The listing builds one solid part. Answer for the finished solid, in the listing's coordinates (mm). A direction names the side the tool comes from. Round coordinates to 2 decimals unless told otherwise and drop trailing zeros. Write each loop counter-clockwise with the first axis right and the second up, starting at its lowest first coordinate (ties: lowest second). Pieces come first, ordered by that corner, then holes.
Autodesk Inventor part; units mm, degrees
ref_plane "YZ Plane" through (0, 0, 0) normal (1, 0, 0) x (0, 1, 0)
ref_plane "XZ Plane" through (0, 0, 0) normal (0, 1, 0) x (-1, 0, 0)
ref_plane "XY Plane" through (0, 0, 0) normal (0, 0, 1) x (1, 0, 0)
sketch "Sketch4" plane through (0, 0, 0) normal (0, 0, 1) x (1, 0, 0)
  line L0 (0, 0) -> (0, 60.2234)
  line L1 (0, 60.2234) -> (25.4, 60.2234)
  line L2 (25.4, 60.2234) -> (25.4, 53.8734)
  line L3 (25.4, 53.8734) -> (0, 53.8734)
  line L4 (0, 60.2234) -> (-12.7, 60.2234)
  line L5 (-12.7, 60.2234) -> (-12.7, 0)
  line L6 (-12.7, 0) -> (0, 0)
  dimension "d25" = 60.2234
  dimension "d26" = 6.35
  dimension "d27" = 25.4
  dimension "d28" = 12.7
extrude "Extrusion3" add sketch "Sketch4" along normal blind 25.4
sketch "Sketch5" plane through (-12.7, 60.2234, 0) normal (0, 1, 0) x (1, 0, 0)
  line L0 (38.1, 0) -> (38.1, -25.4)
  line L1 (38.1, -25.4) -> (0, -25.4)
  point P0 (25.4, -12.7)
  point P1 (15.621, -11.3751)
  point P2 (17.5484, -18.678)
  point P3 (24.0751, -22.479)
  point P4 (31.378, -20.5516)
  point P5 (35.179, -14.0249)
  point P6 (33.2516, -6.722)
  point P7 (26.7249, -2.921)
  point P8 (19.422, -4.8484)
  dimension "d36" = 360
  dimension "d45" = 9.779
  dimension "d46" = 12.7
  dimension "d47" = 12.7
hole "Hole2" at (2.921, 60.2234, 11.3751) at (4.8484, 60.2234, 18.678) at (11.3751, 60.2234, 22.479) at (18.678, 60.2234, 20.5516) at (22.479, 60.2234, 14.0249) at (20.5516, 60.2234, 6.722) at (14.0249, 60.2234, 2.921) at (6.722, 60.2234, 4.8484) direction (0, -1, 0) diameter 2.7178 end through all
properties part number "wheel arm stand off"
1. Straight lines are drawn through the part: line 1 along X through (y, z) = (20.5, 10); line 2 along Y through (x, z) = (4, 4.75). For each, find the intervals that lie inside material, in ascending order.
Geometry says:
line 1: x = -12.7 to 0
line 2: y = 53.87 to 60.22
2. For a pull along Z with two mould halves and no side action, classify faces 1 (the face through (19.204, 57.004, 6.545)), 2 (the face through (25.4, 57, 13)), 3 (the face through (-2, 37, 25.4)) as released by +Z, released by -Z, zero draft, split by the parting line, or undercut.
Geometry says:
face 1: undercut
face 2: zero draft
face 3: released by +Z
3. A tool of negligible diameter and unlimited length cuts with its end or side. For faces 4 (the face through (15.351, 57.004, 2.626)), 5 (the face through (0, 27, 13)), from which of +Z, -Z, +X, -X, +Y, -Y can it reach the whole face along a straight path? Write none if from no direction.
Geometry says:
face 4: +Y, -Y
face 5: +Z, -Z, +X, -Y
4. Section B-B on z = 8.75 is taken. Determine the outline of the cut face in (x, y).
Geometry says:
outline: (-12.7, 0) - (0, 0) - (0, 53.87) - (25.4, 53.87) - (25.4, 60.22) - (-12.7, 60.22) - close
5. Given pin 1 (3 mm diameter, centred on x = 11.38, z = 22.48, fed in from -Y); pin 2 (3 mm diameter, centred on y = 41, z = 19, fed in from +X), each flat-ended and moving along its own axis, determine where each tip first touches the part or whether it passes through.
Geometry says:
pin 1: stops at y = 53.87
pin 2: stops at x = 0
6. Section C-C on y = 29 is taken. Determine the outline of the cut face in (x, z), plus the area to 3 significant figures.
Geometry says:
outline: (-12.7, 0) - (0, 0) - (0, 25.4) - (-12.7, 25.4) - close
area: 323 mm2
7. Section A-A on z = 14.25 is taken. Determine the outline of the cut face in (x, y), plus the area to 3 significant figures.
Geometry says:
outline: (-12.7, 0) - (0, 0) - (0, 53.87) - (21.14, 53.87) - (21.14, 60.22) - (-12.7, 60.22) - close; (23.82, 53.87) - (25.4, 53.87) - (25.4, 60.22) - (23.82, 60.22) - close
area: 909 mm2
8. Section D-D on x = 16 is taken. Determine the outline of the cut face in (y, z).
Geometry says:
outline: (53.87, 0) - (60.22, 0) - (60.22, 25.4) - (53.87, 25.4) - close
